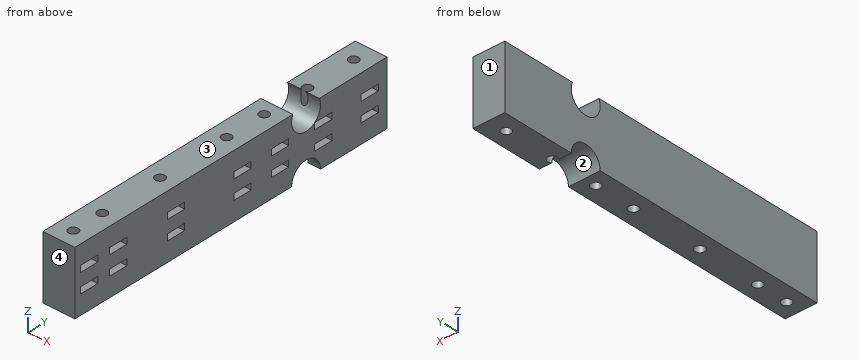
from build123d import *

# Parameters (mm, degrees)
BOX183_W          = 16
BOX183_H          = 6
BOX183_DEPTH      = 2
BOX184_W          = 16
BOX184_H          = 6
BOX184_DEPTH      = 2
BOX185_W          = 16
BOX185_H          = 6
BOX185_DEPTH      = 2
BOX186_W          = 16
BOX186_H          = 6
BOX186_DEPTH      = 2
BOX187_W          = 16
BOX187_H          = 6
BOX187_DEPTH      = 2
BOX188_W          = 16
BOX188_H          = 6
BOX188_DEPTH      = 2
BOX189_W          = 16
BOX189_H          = 6
BOX189_DEPTH      = 2
BOX190_W          = 16
BOX190_H          = 6
BOX190_DEPTH      = 2
BOX191_W          = 16
BOX191_H          = 6
BOX191_DEPTH      = 2
BOX192_W          = 16
BOX192_H          = 6
BOX192_DEPTH      = 2
BOX193_W          = 16
BOX193_H          = 6
BOX193_DEPTH      = 2
BOX194_W          = 16
BOX194_H          = 6
BOX194_DEPTH      = 2
BOX195_W          = 16
BOX195_H          = 6
BOX195_DEPTH      = 2
BOX182_W          = 16
BOX182_H          = 6
BOX182_DEPTH      = 2
CYLINDER440_R     = 1.5
CYLINDER440_DEPTH = 50
CYLINDER441_R     = 1.5
CYLINDER441_DEPTH = 50
CYLINDER442_R     = 1.5
CYLINDER442_DEPTH = 50
CYLINDER443_R     = 1.5
CYLINDER443_DEPTH = 50
CYLINDER444_R     = 1.5
CYLINDER444_DEPTH = 50
CYLINDER445_R     = 1.5
CYLINDER445_DEPTH = 50
CYLINDER439_R     = 1.5
CYLINDER439_DEPTH = 50
CYLINDER432_R     = 5
CYLINDER432_DEPTH = 100
CYLINDER433_R     = 5
CYLINDER433_DEPTH = 100
CYLINDER434_R     = 5
CYLINDER434_DEPTH = 100
CYLINDER435_R     = 5
CYLINDER435_DEPTH = 100
CYLINDER436_R     = 5
CYLINDER436_DEPTH = 100
CYLINDER437_R     = 5
CYLINDER437_DEPTH = 100
CYLINDER438_R     = 5
CYLINDER438_DEPTH = 100
CYLINDER431_R     = 5
CYLINDER431_DEPTH = 100
BOX181_W          = 10
BOX181_H          = 108
BOX181_DEPTH      = 20


with BuildPart() as krychle183:
    # Box183 → Box183 (new body)
    with BuildSketch(Plane(origin=(60, 2, 16), x_dir=(1, 0, 0), z_dir=(0, 0, 1))):
        with Locations((8, 3)):
            Rectangle(BOX183_W, BOX183_H)
    extrude(amount=BOX183_DEPTH)


with BuildPart() as krychle184:
    # Box184 → Box184 (new body)
    with BuildSketch(Plane(origin=(60, -21, 10), x_dir=(1, 0, 0), z_dir=(0, 0, 1))):
        with Locations((8, 3)):
            Rectangle(BOX184_W, BOX184_H)
    extrude(amount=BOX184_DEPTH)


with BuildPart() as krychle185:
    # Box185 → Box185 (new body)
    with BuildSketch(Plane(origin=(60, -21, 16), x_dir=(1, 0, 0), z_dir=(0, 0, 1))):
        with Locations((8, 3)):
            Rectangle(BOX185_W, BOX185_H)
    extrude(amount=BOX185_DEPTH)


with BuildPart() as krychle186:
    # Box186 → Box186 (new body)
    with BuildSketch(Plane(origin=(60, -41, 10), x_dir=(1, 0, 0), z_dir=(0, 0, 1))):
        with Locations((8, 3)):
            Rectangle(BOX186_W, BOX186_H)
    extrude(amount=BOX186_DEPTH)


with BuildPart() as krychle187:
    # Box187 → Box187 (new body)
    with BuildSketch(Plane(origin=(60, -41, 16), x_dir=(1, 0, 0), z_dir=(0, 0, 1))):
        with Locations((8, 3)):
            Rectangle(BOX187_W, BOX187_H)
    extrude(amount=BOX187_DEPTH)


with BuildPart() as krychle188:
    # Box188 → Box188 (new body)
    with BuildSketch(Plane(origin=(60, -51, 10), x_dir=(1, 0, 0), z_dir=(0, 0, 1))):
        with Locations((8, 3)):
            Rectangle(BOX188_W, BOX188_H)
    extrude(amount=BOX188_DEPTH)


with BuildPart() as krychle189:
    # Box189 → Box189 (new body)
    with BuildSketch(Plane(origin=(60, -51, 16), x_dir=(1, 0, 0), z_dir=(0, 0, 1))):
        with Locations((8, 3)):
            Rectangle(BOX189_W, BOX189_H)
    extrude(amount=BOX189_DEPTH)


with BuildPart() as krychle190:
    # Box190 → Box190 (new body)
    with BuildSketch(Plane(origin=(60, 15, 10), x_dir=(1, 0, 0), z_dir=(0, 0, 1))):
        with Locations((8, 3)):
            Rectangle(BOX190_W, BOX190_H)
    extrude(amount=BOX190_DEPTH)


with BuildPart() as krychle191:
    # Box191 → Box191 (new body)
    with BuildSketch(Plane(origin=(60, 30, 10), x_dir=(1, 0, 0), z_dir=(0, 0, 1))):
        with Locations((8, 3)):
            Rectangle(BOX191_W, BOX191_H)
    extrude(amount=BOX191_DEPTH)


with BuildPart() as krychle192:
    # Box192 → Box192 (new body)
    with BuildSketch(Plane(origin=(60, 46, 10), x_dir=(1, 0, 0), z_dir=(0, 0, 1))):
        with Locations((8, 3)):
            Rectangle(BOX192_W, BOX192_H)
    extrude(amount=BOX192_DEPTH)


with BuildPart() as krychle193:
    # Box193 → Box193 (new body)
    with BuildSketch(Plane(origin=(60, 15, 16), x_dir=(1, 0, 0), z_dir=(0, 0, 1))):
        with Locations((8, 3)):
            Rectangle(BOX193_W, BOX193_H)
    extrude(amount=BOX193_DEPTH)


with BuildPart() as krychle194:
    # Box194 → Box194 (new body)
    with BuildSketch(Plane(origin=(60, 30, 16), x_dir=(1, 0, 0), z_dir=(0, 0, 1))):
        with Locations((8, 3)):
            Rectangle(BOX194_W, BOX194_H)
    extrude(amount=BOX194_DEPTH)


with BuildPart() as krychle195:
    # Box195 → Box195 (new body)
    with BuildSketch(Plane(origin=(60, 46, 16), x_dir=(1, 0, 0), z_dir=(0, 0, 1))):
        with Locations((8, 3)):
            Rectangle(BOX195_W, BOX195_H)
    extrude(amount=BOX195_DEPTH)


with BuildPart() as compound585:
    # Box182 → Box182 (new body)
    with BuildSketch(Plane(origin=(60, 2, 10), x_dir=(1, 0, 0), z_dir=(0, 0, 1))):
        with Locations((8, 3)):
            Rectangle(BOX182_W, BOX182_H)
    extrude(amount=BOX182_DEPTH)

    # Compound585: union Krychle183, Krychle184, Krychle185, Krychle186, Krychle187, Krychle188, Krychle189, Krychle190, Krychle191, Krychle192, Krychle193, Krychle194, Krychle195
    add(krychle183.part)
    add(krychle184.part)
    add(krychle185.part)
    add(krychle186.part)
    add(krychle187.part)
    add(krychle188.part)
    add(krychle189.part)
    add(krychle190.part)
    add(krychle191.part)
    add(krychle192.part)
    add(krychle193.part)
    add(krychle194.part)
    add(krychle195.part)


with BuildPart() as compound585_1:
    # Compound585 placement: moved
    add(compound585.part.moved(Location((39, 24, 3))))


with BuildPart() as obj1:
    # Cylinder440 → Cylinder440 (new body)
    with BuildSketch(Plane(origin=(63, -18, -12), x_dir=(1, 0, 0), z_dir=(0, 0, 1))):
        Circle(CYLINDER440_R)
    extrude(amount=CYLINDER440_DEPTH)


with BuildPart() as obj2:
    # Cylinder441 → Cylinder441 (new body)
    with BuildSketch(Plane(origin=(63, -38, -12), x_dir=(1, 0, 0), z_dir=(0, 0, 1))):
        Circle(CYLINDER441_R)
    extrude(amount=CYLINDER441_DEPTH)


with BuildPart() as obj3:
    # Cylinder442 → Cylinder442 (new body)
    with BuildSketch(Plane(origin=(63, -48, -12), x_dir=(1, 0, 0), z_dir=(0, 0, 1))):
        Circle(CYLINDER442_R)
    extrude(amount=CYLINDER442_DEPTH)


with BuildPart() as obj4:
    # Cylinder443 → Cylinder443 (new body)
    with BuildSketch(Plane(origin=(63, 18, -12), x_dir=(1, 0, 0), z_dir=(0, 0, 1))):
        Circle(CYLINDER443_R)
    extrude(amount=CYLINDER443_DEPTH)


with BuildPart() as obj5:
    # Cylinder444 → Cylinder444 (new body)
    with BuildSketch(Plane(origin=(63, 33, -12), x_dir=(1, 0, 0), z_dir=(0, 0, 1))):
        Circle(CYLINDER444_R)
    extrude(amount=CYLINDER444_DEPTH)


with BuildPart() as obj6:
    # Cylinder445 → Cylinder445 (new body)
    with BuildSketch(Plane(origin=(63, 49, -12), x_dir=(1, 0, 0), z_dir=(0, 0, 1))):
        Circle(CYLINDER445_R)
    extrude(amount=CYLINDER445_DEPTH)


with BuildPart() as compound590:
    # Cylinder439 → Cylinder439 (new body)
    with BuildSketch(Plane(origin=(63, 5, -12), x_dir=(1, 0, 0), z_dir=(0, 0, 1))):
        Circle(CYLINDER439_R)
    extrude(amount=CYLINDER439_DEPTH)

    # Compound590: union obj1, obj2, obj3, obj4, obj5, obj6
    add(obj1.part)
    add(obj2.part)
    add(obj3.part)
    add(obj4.part)
    add(obj5.part)
    add(obj6.part)


with BuildPart() as compound590_1:
    # Compound590 placement: moved
    add(compound590.part.moved(Location((39, 24, 0))))


with BuildPart() as obj7:
    # Cylinder432 → Cylinder432 (new body)
    with BuildSketch(Plane(origin=(24, -51, 25), x_dir=(0, 0, -1), z_dir=(1, 0, 0))):
        Circle(CYLINDER432_R)
    extrude(amount=CYLINDER432_DEPTH)


with BuildPart() as obj8:
    # Cylinder433 → Cylinder433 (new body)
    with BuildSketch(Plane(origin=(24, 36, 34), x_dir=(0, 0, -1), z_dir=(1, 0, 0))):
        Circle(CYLINDER433_R)
    extrude(amount=CYLINDER433_DEPTH)


with BuildPart() as obj9:
    # Cylinder434 → Cylinder434 (new body)
    with BuildSketch(Plane(origin=(24, -36, 34), x_dir=(0, 0, -1), z_dir=(1, 0, 0))):
        Circle(CYLINDER434_R)
    extrude(amount=CYLINDER434_DEPTH)


with BuildPart() as obj10:
    # Cylinder435 → Cylinder435 (new body)
    with BuildSketch(Plane(origin=(24, -23, -5), x_dir=(0, 0, -1), z_dir=(1, 0, 0))):
        Circle(CYLINDER435_R)
    extrude(amount=CYLINDER435_DEPTH)


with BuildPart() as obj11:
    # Cylinder436 → Cylinder436 (new body)
    with BuildSketch(Plane(origin=(24, 51, 7), x_dir=(0, 0, -1), z_dir=(1, 0, 0))):
        Circle(CYLINDER436_R)
    extrude(amount=CYLINDER436_DEPTH)


with BuildPart() as obj12:
    # Cylinder437 → Cylinder437 (new body)
    with BuildSketch(Plane(origin=(24, 23, -5), x_dir=(0, 0, -1), z_dir=(1, 0, 0))):
        Circle(CYLINDER437_R)
    extrude(amount=CYLINDER437_DEPTH)


with BuildPart() as obj13:
    # Cylinder438 → Cylinder438 (new body)
    with BuildSketch(Plane(origin=(24, -51, 7), x_dir=(0, 0, -1), z_dir=(1, 0, 0))):
        Circle(CYLINDER438_R)
    extrude(amount=CYLINDER438_DEPTH)


with BuildPart() as compound589:
    # Cylinder431 → Cylinder431 (new body)
    with BuildSketch(Plane(origin=(24, 51, 25), x_dir=(0, 0, -1), z_dir=(1, 0, 0))):
        Circle(CYLINDER431_R)
    extrude(amount=CYLINDER431_DEPTH)

    # Compound589: union obj7, obj8, obj9, obj10, obj11, obj12, obj13
    add(obj7.part)
    add(obj8.part)
    add(obj9.part)
    add(obj10.part)
    add(obj11.part)
    add(obj12.part)
    add(obj13.part)


with BuildPart() as compound589_1:
    # Compound589 placement: moved
    add(compound589.part.moved(Location((32, 0, 0))))


with BuildPart() as cut365:
    # Box181 → Box181 (new body)
    with BuildSketch(Plane(origin=(97, -29, 7), x_dir=(1, 0, 0), z_dir=(0, 0, 1))):
        with Locations((5, 54)):
            Rectangle(BOX181_W, BOX181_H)
    extrude(amount=BOX181_DEPTH)

    # Cut363: cut Compound589
    add(compound589_1.part, mode=Mode.SUBTRACT)

    # Cut364: cut Compound590
    add(compound590_1.part, mode=Mode.SUBTRACT)

    # Cut365: cut Compound585
    add(compound585_1.part, mode=Mode.SUBTRACT)


solid = cut365.part
Read the model definition and answer for the solid it produces. Units are mm, in the model's axes. Face numbers are marked on the shaded views. Round coordinates to 2 decimals unless told otherwise and drop trailing zeros. Write each loop counter-clockwise with the first axis right and the second up, starting at its lowest first coordinate (ties: lowest second). Pieces come first, ordered by that corner, then holes.
Q1. The mould has two halves that part along Y. Classify the marked faces 1, 2, 3 and 4: released by +Y, released by -Y, zero draft, split by the parting line, or undercut.
Values:
face 1: released by +Y
face 2: undercut
face 3: zero draft
face 4: released by -Y
Q2. Find section B-B on x = 98. Determine the outline of the cut face in (y, z), and give its area (3 significant figures).
Values:
outline: (-29, 7) - (46, 7) arc R5 cw to (56, 7) - (79, 7) - (79, 27) - (55.58, 27) arc R5 cw (long way) to (46.42, 27) - (-29, 27) - close
area: 2,060 mm2
Q3. Straight lines are drawn through the part: line 1 (Z direction, x = 101.5, y = 7.5); line 2 (X direction, y = 73, z = 23.4); line 3 (Y direction, x = 98.25, z = 26). For each, find the intervals that lie inside material, in ascending order.
Values:
line 1: z = 7 to 13, 15 to 19, 21 to 27
line 2: x = 97 to 100.5, 103.5 to 107
line 3: y = -29 to 46.1, 55.9 to 79
Q4. Find section A-A on y = 57. Determine the outline of the cut face in (x, z), and give its area (3 significant figures).
Values:
outline: (97, 7) - (100.5, 7) - (100.5, 13) - (99, 13) - (99, 15) - (100.5, 15) - (100.5, 19) - (99, 19) - (99, 21) - (100.5, 21) - (100.5, 27) - (97, 27) - close; (103.5, 7) - (107, 7) - (107, 13) - (103.5, 13) - close; (103.5, 15) - (107, 15) - (107, 19) - (103.5, 19) - close; (103.5, 21) - (107, 21) - (107, 27) - (103.5, 27) - close
area: 120 mm2
Q5. Flat-ended cylindrical pins translate along their axes: P1, Ø2.5, axis at x = 102, y = -14, coming from the +Z side; P2, Ø0.6, axis at y = 58, z = 20.5, coming from the +X side. Find the tip coordinate at first contact, or state that the pin passes through.
Values:
P1: passes through
P2: stops at x = 99
